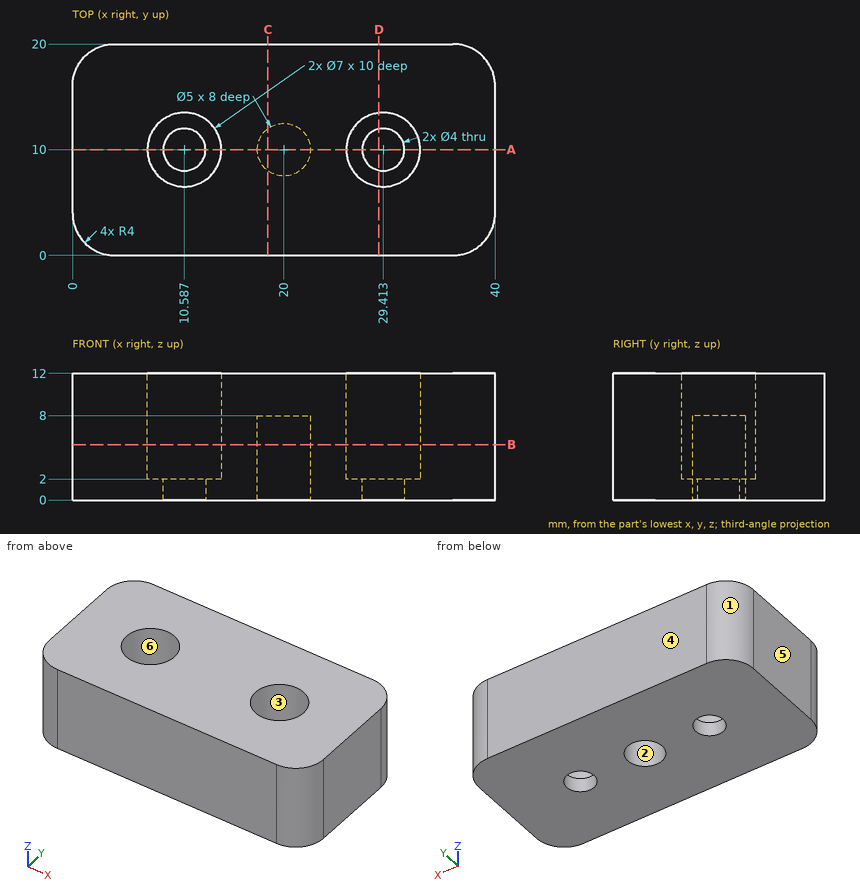
Design review of the part shown in the three views and the two pictorial views. Dimensions are in mm from the part's minimum x, y and z. A direction names the side the tool comes from. Coordinates: 2 decimals unless noted, no trailing zeros. Write each loop counter-clockwise with the first axis right and the second up, starting at its lowest first coordinate (ties: lowest second). Pieces come first, ordered by that corner, then holes.
(1) Add section A-A on y = 10. Give the boundary of the cut face in (x, z).
(2) For pin 1 Ø6.5 at (x, y) = (29.41, 10) entering from +Z; pin 2 Ø2.5 at (x, y) = (19.5, 9) entering from -Z; pin 3 Ø3 at (x, y) = (29.41, 10) entering from +Z, all flat-tipped, find the tip position at first contact; note any pin that passes through.
(3) The part is to be moulded in two halves that separate along Y. For the marked faces 4, 5 and 6, say which applies: +Y half, -Y half, draft (parallel to the pull), parting line (faces both ways), or undercut.
(4) Tool access review of the marked faces 1, 2 and 3: name each direction out of +Z, -Z, +X, -X, +Y, -Y from which nothing blocks a thin tool from reaching the whole face with its end or side.
(5) Wall thickness on probe 1 along Y at (x, z) = (20, 6); probe 2 along Y at (x, z) = (18, 4); probe 3 along X at (y, z) = (17.75, 2): over which ranges is each line inside the solid? List them lowest first.
(6) Add section C-C on x = 18.5. Give the boundary of the cut face in (y, z), then the cut area to 3 significant figures.
(7) Add section B-B on z = 5.25. Give the boundary of the cut face in (x, y).
(8) Add section D-D on x = 29. Give the boundary of the cut face in (y, z) (1 decimal), then the cut area to 3 significant figures.
Answer sheet:
1. outline: (0, 0) - (8.59, 0) - (8.59, 2) - (7.09, 2) - (7.09, 12) - (0, 12) - close; (12.59, 0) - (17.5, 0) - (17.5, 8) - (22.5, 8) - (22.5, 0) - (27.41, 0) - (27.41, 2) - (25.91, 2) - (25.91, 12) - (14.09, 12) - (14.09, 2) - (12.59, 2) - close; (31.41, 0) - (40, 0) - (40, 12) - (32.91, 12) - (32.91, 2) - (31.41, 2) - close
2. pin 1: stops at z = 2
2. pin 2: stops at z = 8
2. pin 3: passes through
3. face 4: +Y half
3. face 5: draft
3. face 6: undercut
4. face 1: +Z, -Z, -X, +Y
4. face 2: -Z
4. face 3: +Z
5. probe 1: y = 0 to 7.5, 12.5 to 20
5. probe 2: y = 0 to 8.5, 11.5 to 20
5. probe 3: x = 0.4 to 39.6
6. outline: (0, 0) - (8, 0) - (8, 8) - (12, 8) - (12, 0) - (20, 0) - (20, 12) - (0, 12) - close
6. area: 208 mm2
7. outline: (0, 4) arc R4 ccw to (4, 0) - (36, 0) arc R4 ccw to (40, 4) - (40, 16) arc R4 ccw to (36, 20) - (4, 20) arc R4 ccw to (0, 16) - close; hole circle Ø7 at (10.59, 10); hole circle Ø5 at (20, 10); hole circle Ø7 at (29.41, 10)
8. outline: (0, 0) - (8, 0) - (8, 2) - (6.5, 2) - (6.5, 12) - (0, 12) - close; (12, 0) - (20, 0) - (20, 12) - (13.5, 12) - (13.5, 2) - (12, 2) - close
8. area: 163 mm2
